Check sheet for the modelled part. Datum: model origin and axes. Units: mm. Give positions to 0.01 mm unless a question says otherwise; leave off trailing zeros. Loops run counter-clockwise (first coordinate to the right, second up) from the corner with the lowest first, then second, coordinate; pieces in that order, holes last. Notation, with made-up numbers: (-1, 66.25) -> (55, 66.25) arc R10 ccw to (55, 73.25) -> close; hole circle Ø4 at (59, 38.25). An arc over 180 degrees is marked (long way). Write each question's results on one line, items separated by ' | '. Start each with the question number.
1. Cross-section at B-B on y = -12.7. Record the boundary of the cut face in (x, z).
2. Gauge pin test, flat end, axial feed: pin 1 Ø3 at (x, y) = (-35.5, -11.5) entering from +Z. Record the tip position at first contact, or that the pin passes through.
3. Cross-section at D-D on y = -23.75. Record the boundary of the cut face in (x, z), and give its area (3 significant figures).
4. Material ranges on L1, parallel to Z at x = 20.5, y = -12.7; L2, parallel to Z at x = 8.5, y = -12; L3, parallel to Z at x = 43.5, y = -2.5, recorded low to high. Write a range as from..to.
5. Mould release check, pull along Y, two halves, no side actions. Record for faces 1 (the face through (-48.394, -13, -5)), 2 (the face through (0.678, -15.723, 8.497)), 3 (the face through (43.163, -11.198, 34.153)), 4 (the face through (-1, -25.4, 0)): +Y half, -Y half, draft (parallel to the pull), parting line (faces both ways), or undercut.
6. Cross-section at A-A on z = 0. Record the boundary of the cut face in (x, y).
7. Cross-section at C-C on x = 13.5. Record the boundary of the cut face in (y, z).
from build123d import *

# Parameters (mm, degrees)
F0_W     = 96.787006
F0_H     = 43.260872
F6_DEPTH = 25.4
F1_R     = 5
F2_DEPTH = 25.4
F7_R     = 3.81
F8_DEPTH = 96.788006


with BuildPart() as f6:
    # F0 (on Front) → F6 (new body)
    with BuildSketch(Plane.XZ):
        Rectangle(F0_W, F0_H)
    extrude(amount=F6_DEPTH)

    # F1 (on face) → F2 (join)
    with BuildSketch(Plane.XY.offset(21.630436)):
        with Locations((38.393503, -12.7)):
            Circle(F1_R)
    extrude(amount=F2_DEPTH)

    # F7 (on face) → F8 (cut, through all)
    with BuildSketch(Plane.YZ.offset(48.393503)):
        with Locations((-12.7, 10.815218)):
            Circle(F7_R)
        with Locations((-12.7, 0)):
            Circle(F7_R)
        with Locations((-12.7, -10.815218)):
            Circle(F7_R)
    extrude(amount=-F8_DEPTH, mode=Mode.SUBTRACT)


solid = f6.part
Geometry says:
1) outline: (-48.39, -21.63) -> (48.39, -21.63) -> (48.39, -14.63) -> (-48.39, -14.63) -> close; (-48.39, -7.01) -> (48.39, -7.01) -> (48.39, -3.81) -> (-48.39, -3.81) -> close; (-48.39, 3.81) -> (48.39, 3.81) -> (48.39, 7.01) -> (-48.39, 7.01) -> close; (-48.39, 14.63) -> (48.39, 14.63) -> (48.39, 21.63) -> (43.39, 21.63) -> (43.39, 47.03) -> (33.39, 47.03) -> (33.39, 21.63) -> (-48.39, 21.63) -> close
2) pin 1: z = 21.63
3) outline: (-48.39, -21.63) -> (48.39, -21.63) -> (48.39, 21.63) -> (-48.39, 21.63) -> close | area: 4,190 mm^2
4) L1: -21.63..-14.63, -7.01..-3.81, 3.81..7.01, 14.63..21.63 | L2: -21.63..-14.56, -7.07..-3.75, 3.75..7.07, 14.56..21.63 | L3: -21.63..21.63
5) face 1: draft | face 2: undercut | face 3: parting line | face 4: -Y half
6) outline: (-48.39, -25.4) -> (48.39, -25.4) -> (48.39, -16.51) -> (-48.39, -16.51) -> close; (-48.39, -8.89) -> (48.39, -8.89) -> (48.39, 0) -> (-48.39, 0) -> close
7) outline: (-25.4, -21.63) -> (0, -21.63) -> (0, 21.63) -> (-25.4, 21.63) -> close; hole circle Ø7.62 at (-12.7, -10.82); hole circle Ø7.62 at (-12.7, 0); hole circle Ø7.62 at (-12.7, 10.82)
